```python
from build123d import *


with BuildPart() as part:
    # Sketch1 → Revolve2 (revolve)
    with BuildSketch(Plane(origin=(0, 0, 0), x_dir=(0, 0, -1), z_dir=(1, 0, 0))):
        Polygon((-85, 25), (85, 25), (85, 29.115175046), (55.901270972, 29.115175046), (55.901270972, 43.144153468), (53.901270972, 43.144153468), (53.901270972, 41.530001869), (44.901270972, 41.530001869), (44.901270972, 43.144153468), (42.901270972, 43.144153468), (42.901270972, 29.961940535), (6.5, 29.961940535), (6.5, 43.144153468), (4.5, 43.144153468), (4.5, 41.530001869), (-4.5, 41.530001869), (-4.5, 43.144153468), (-6.5, 43.144153468), (-6.5, 30.363940149), (-45.552167267, 30.363940149), (-45.552167267, 43.144153468), (-47.552167267, 43.144153468), (-47.552167267, 41.530001869), (-56.552167267, 41.530001869), (-56.552167267, 43.144153468), (-58.552167267, 43.144153468), (-58.552167267, 30.363940149), (-85, 30.363940149), align=None)
    revolve(axis=Axis((0, 0, 119.060774984), (0, 0, -1)))


solid = part.part
```
For this review, take the finished solid that the model builds, in its own axes (mm). A direction names the side the tool comes from. Coordinates: 2 decimals unless noted, no trailing zeros. Order: outer loops, then holes, each group sorted by start corner. A loop starts at its lowest first (then second) coordinate and runs counter-clockwise, first axis right, second up. Notation, with made-up numbers: (-31.75, 29) - (7.25, 29) arc R29 ccw to (7.25, 52) - close; hole circle Ø1 at (39, 42.25). An arc over 180 degrees is marked (long way). Answer as a JSON object with one key per item and string values. Group by question number.
1. We need section A-A on z = 12. State the section outline as (x, y) points.
2. We need section B-B on y = 33. Give the number of separate pieces and of enclosed holes in the cut face, then the cut area to 3 significant figures.
3. For faces 1 (the cylindrical face through (12.96, 41.15, 57.57)), 2 (the cylindrical face through (-11.151, 26.895, -70.247)), 3 (the cylindrical face through (-29.642, -6.582, 71.961)), 4 (the cylindrical face through (-29.642, -6.582, 26.299)), list the 3-axis set-ups (+Z, -Z, +X, -X, +Y, -Y) from which the entire face can be reached by the end or side of a thin tool; tool diameter is ignored.
4. The part is to be moulded in two halves that separate along Z. For faces 5 (the flat face through (25, 4, 85)), 6 (the cylindrical face through (12.96, 41.15, -43.89)), 7 (the cylindrical face through (-25.27, -32.957, 0.063)), 8 (the cylindrical face through (-25.27, -32.957, -49.338)), say which applies: pulls with the +Z half, pulls with the -Z half, needs draft (parallel to the pull), parting line crosses it, or undercut.
5. Clearance check with flat-ended pins moving along their axes: P1, Ø1.5, axis at x = -1, z = 65, coming from the -Y side; P2, Ø10, axis at y = -33, z = -6.5, coming from the +X side; P3, Ø1.5, axis at y = 18.5, z = -11.5, coming from the +X side. State where each tip first meets the part, or that it passes through.
6. For probe 1 along Z at (x, y) = (28.5, -17.5); probe 2 along Z at (x, y) = (26.5, 33); probe 3 along X at (y, z) = (0, -51), list the stretches that pass through material, from the lowest coordinate up.
Final values:
{
 "1": {"outline": "circle Ø60.73 at (0, 0); hole circle Ø50 at (0, 0)"},
 "2": {"separate pieces": "3", "enclosed holes": "0", "area": "2,030 mm²"},
 "3": {"face 1": "+Z, -Z", "face 2": "-Z", "face 3": "+Z", "face 4": "none"},
 "4": {"face 5": "pulls with the +Z half", "face 6": "needs draft", "face 7": "undercut", "face 8": "undercut"},
 "5": {"P1": "y = -30.36", "P2": "x = 32.82", "P3": "x = 24.14"},
 "6": {"probe 1": "-55.9 to -42.9, -6.5 to 6.5, 45.55 to 58.55", "probe 2": "-55.9 to -53.9, -44.9 to -42.9, -6.5 to -4.5, 4.5 to 6.5, 45.55 to 47.55, 56.55 to 58.55", "probe 3": "-41.53 to -25, 25 to 41.53"}
}
